Work out the finished part from the listing and answer in its coordinate system (mm). A direction names the side the tool comes from. Coordinates: 2 decimals unless noted, no trailing zeros. Order: outer loops, then holes, each group sorted by start corner. A loop starts at its lowest first (then second) coordinate and runs counter-clockwise, first axis right, second up. Notation, with made-up numbers: (-31.5, 73) - (13.5, 73) arc R19 ccw to (13.5, 92) - close; hole circle Ø6 at (75, -7.5). An arc over 180 degrees is marked (long way). Answer as a JSON object with one key per item and string values. Group by question number.
1) Each of these flat-tipped pins is pushed along its axis until it touches: P1, Ø1.8, axis at x = 29.5, z = -12.5, coming from the +Y side; P2, Ø1.1, axis at y = 2, z = -11, coming from the +X side; P3, Ø3.5, axis at x = -23.5, z = 5, coming from the +Y side; P4, Ø1.5, axis at x = -23.5, y = 1.5, coming from the +Z side. Where does it stop, or does it pass through?
2) Section D-D (z = -12.5) is taken. Give the vertices of the cut face in (x, y), plus the area to 3 significant figures.
3) Section A-A (z = -5) is taken. Give the vertices of the cut face in (x, y).
4) Section B-B (x = -8.5) is taken. Give the vertices of the cut face in (y, z).
5) Section C-C (y = 2.25) is taken. Count the separate pieces of the cut face and the enclosed holes in it, plus the area to 3 significant figures.
6) Find the intervals of material crossed by line 1 along X through (y, z) = (1.45, -5); line 2 along X through (y, z) = (1.3, -12.5); line 3 along X through (y, z) = (3.2, 11.5), in increasing order.
7) A tool of negligible diameter and unlimited length cuts with its end or side. For faces 1 (the face through (-14, 2, 8.5)), 2 (the face through (32.719, 1.521, 15.094)), 3 (the face through (29.5, 1, 0)), 4 (the face through (-25, 2, 1.5)), 5 (the face through (5.6, 3.5, 10)), from which of +Z, -Z, +X, -X, +Y, -Y can it reach the whole face along a straight path? Write none if from no direction.
from build123d import *

# Parameters (mm, degrees)
SKETCH_1_R          = 1.5
SKETCH_1_W          = 24
SKETCH_1_H          = 15
EXTRUDE_1_DEPTH     = 3
SKETCH_2_R          = 2.5
SKETCH_2_R_2        = 1.5
EXTRUDE_2_DEPTH     = 1
CUT_EXTRUDE_1_REACH = 41.246
SKETCH_3_W          = 7
SKETCH_3_H          = 3
FILLET_1_R          = 8
EXTRUDE_3_DEPTH     = 3
CUT_EXTRUDE_2_REACH = 41.246
SKETCH_5_R          = 1.5
EXTRUDE_START       = -3
SKETCH_6_R          = 1.5
EXTRUDE_4_DEPTH     = 3
CUT_EXTRUDE_3_DEPTH = 40.246018906
FILLET_2_R          = 3


with BuildPart() as part:
    # 草图1 → 凸台-拉伸1 (new body)
    with BuildSketch(Plane(origin=(0, 0, 0), x_dir=(1, 0, 0), z_dir=(0, 1, 0))):
        Polygon((-14, -8.5), (0, -8.5), (0, -17.5), (35, -17.5), (35, 17.5), (0, 17.5), (0, 8.5), (-14, 8.5), (-21, 8.5), (-21, -8.5), align=None)
        with Locations(Location((-2.5, 0, 0), (0, 0, 270))):
            Circle(SKETCH_1_R, mode=Mode.SUBTRACT)
        with Locations(Location((29.5, -12.5, 0), (0, 0, 270))):
            Circle(SKETCH_1_R, mode=Mode.SUBTRACT)
        with Locations(Location((5.5, -12.5, 0), (0, 0, 270))):
            Circle(SKETCH_1_R, mode=Mode.SUBTRACT)
        with Locations(Location((29.5, 12.5, 0), (0, 0, 270))):
            Circle(SKETCH_1_R, mode=Mode.SUBTRACT)
        with Locations(Location((5.5, 12.5, 0), (0, 0, 270))):
            Circle(SKETCH_1_R, mode=Mode.SUBTRACT)
        with Locations(Location((-17.5, -5, 0), (0, 0, 270))):
            Circle(SKETCH_1_R, mode=Mode.SUBTRACT)
        with Locations(Location((-17.5, 5, 0), (0, 0, 270))):
            Circle(SKETCH_1_R, mode=Mode.SUBTRACT)
        with Locations((17.5, 0)):
            Rectangle(SKETCH_1_W, SKETCH_1_H, mode=Mode.SUBTRACT)
    extrude(amount=EXTRUDE_1_DEPTH)

    # 草图2 → 凸台-拉伸2 (add)
    # profile 1 of 4: a face of its own
    with BuildSketch(Plane(origin=(0, 3, 0), x_dir=(1, 0, 0), z_dir=(0, 1, 0))):
        with Locations(Location((5.5, 12.5, 0), (0, 0, 270))):
            Circle(SKETCH_2_R)
        with Locations(Location((5.5, 12.5, 0), (0, 0, 270))):
            Circle(SKETCH_2_R_2, mode=Mode.SUBTRACT)
    # profile 2 of 4: a face of its own
    with BuildSketch(Plane(origin=(0, 3, 0), x_dir=(1, 0, 0), z_dir=(0, 1, 0))):
        with Locations(Location((29.5, 12.5, 0), (0, 0, 270))):
            Circle(SKETCH_2_R)
        with Locations(Location((29.5, 12.5, 0), (0, 0, 270))):
            Circle(SKETCH_2_R_2, mode=Mode.SUBTRACT)
    # profile 3 of 4: a face of its own
    with BuildSketch(Plane(origin=(0, 3, 0), x_dir=(1, 0, 0), z_dir=(0, 1, 0))):
        with Locations(Location((29.5, -12.5, 0), (0, 0, 270))):
            Circle(SKETCH_2_R)
        with Locations(Location((29.5, -12.5, 0), (0, 0, 270))):
            Circle(SKETCH_2_R_2, mode=Mode.SUBTRACT)
    # profile 4 of 4: a face of its own
    with BuildSketch(Plane(origin=(0, 3, 0), x_dir=(1, 0, 0), z_dir=(0, 1, 0))):
        with Locations(Location((5.5, -12.5, 0), (0, 0, 270))):
            Circle(SKETCH_2_R)
        with Locations(Location((5.5, -12.5, 0), (0, 0, 270))):
            Circle(SKETCH_2_R_2, mode=Mode.SUBTRACT)
    extrude(amount=EXTRUDE_2_DEPTH)

    # 草图3 → 切除-拉伸1 (cut, up to next)
    with BuildSketch(Plane(origin=(0, 3, 0), x_dir=(1, 0, 0), z_dir=(0, 1, 0)), mode=Mode.PRIVATE) as cut_extrude_1_sk1:
        with Locations((-17.5, 0)):
            Rectangle(SKETCH_3_W, SKETCH_3_H)
    cut_extrude_1_tool1 = extrude(cut_extrude_1_sk1.sketch, amount=-CUT_EXTRUDE_1_REACH, mode=Mode.PRIVATE) & part.part
    add(cut_extrude_1_tool1.solids().sort_by_distance((-17.5, 3, 0))[0], mode=Mode.SUBTRACT)

    # 圆角1
    fillet_1_edges = [part.edges().sort_by_distance(p)[0] for p in [
        (0, 1.5, -17.5),
        (35, 1.5, -17.5),
        (35, 1.5, 17.5),
        (0, 1.5, 17.5),
    ]]
    fillet(fillet_1_edges, radius=FILLET_1_R)

    # 草图4 → 凸台-拉伸3 (add)
    with BuildSketch(Plane(origin=(0, 3, 0), x_dir=(1, 0, 0), z_dir=(0, 1, 0))):
        Polygon((-21, 8.5), (-27, 8.5), (-27, 1.5), (-22.2, 1.5), (-22.2, -1.5), (-27, -1.5), (-27, -8.5), (-21, -8.5), (-21, -1.5), (-14, -1.5), (-14, 1.5), (-21, 1.5), align=None)
    extrude(amount=-EXTRUDE_3_DEPTH)

    # 草图5 → 切除-拉伸2 (cut, up to next)
    with BuildSketch(Plane(origin=(0, 3, 0), x_dir=(1, 0, 0), z_dir=(0, 1, 0)), mode=Mode.PRIVATE) as cut_extrude_2_sk1:
        with Locations(Location((-23.5, 5, 0), (0, 0, 270))):
            Circle(SKETCH_5_R)
    cut_extrude_2_tool1 = extrude(cut_extrude_2_sk1.sketch, amount=-CUT_EXTRUDE_2_REACH, mode=Mode.PRIVATE) & part.part
    # 草图5 → 切除-拉伸2 (cut, up to next)
    with BuildSketch(Plane(origin=(0, 3, 0), x_dir=(1, 0, 0), z_dir=(0, 1, 0)), mode=Mode.PRIVATE) as cut_extrude_2_sk2:
        with Locations(Location((-23.5, -5, 0), (0, 0, 270))):
            Circle(SKETCH_5_R)
    cut_extrude_2_tool2 = extrude(cut_extrude_2_sk2.sketch, amount=-CUT_EXTRUDE_2_REACH, mode=Mode.PRIVATE) & part.part
    # 草图5 → 切除-拉伸2 (cut, up to next)
    with BuildSketch(Plane(origin=(0, 3, 0), x_dir=(1, 0, 0), z_dir=(0, 1, 0)), mode=Mode.PRIVATE) as cut_extrude_2_sk3:
        with Locations(Location((-8.5, 0, 0), (0, 0, 270))):
            Circle(SKETCH_5_R)
    cut_extrude_2_tool3 = extrude(cut_extrude_2_sk3.sketch, amount=-CUT_EXTRUDE_2_REACH, mode=Mode.PRIVATE) & part.part
    add(cut_extrude_2_tool1.solids().sort_by_distance((-23.5, 3, -5))[0], mode=Mode.SUBTRACT)
    add(cut_extrude_2_tool2.solids().sort_by_distance((-23.5, 3, 5))[0], mode=Mode.SUBTRACT)
    add(cut_extrude_2_tool3.solids().sort_by_distance((-8.5, 3, 0))[0], mode=Mode.SUBTRACT)

    # 草图6 → 凸台-拉伸4 (add)
    with BuildSketch(Plane(origin=(0, 3, 0), x_dir=(1, 0, 0), z_dir=(0, 1, 0)).offset(EXTRUDE_START)):
        with Locations((-17.5, 5)):
            Circle(SKETCH_6_R)
        with Locations((-2.5, 0)):
            Circle(SKETCH_6_R)
        with Locations((-17.5, -5)):
            Circle(SKETCH_6_R)
    extrude(amount=EXTRUDE_4_DEPTH)

    # 草图7 → 切除-拉伸3 (cut, through all)
    with BuildSketch(Plane(origin=(0, 3, 0), x_dir=(1, 0, 0), z_dir=(0, 1, 0))):
        Polygon((17.5, 11.5), (12.5, 11.5), (12.5, 7.5), (22.5, 7.5), (22.5, 11.5), align=None)
        Polygon((22.5, -11.5), (17.5, -11.5), (12.5, -11.5), (12.5, -7.5), (22.5, -7.5), align=None)
    extrude(amount=-CUT_EXTRUDE_3_DEPTH, mode=Mode.SUBTRACT)

    # 圆角2
    fillet_2_edges = [part.edges().sort_by_distance(p)[0] for p in [
        (22.5, 1.5, -7.5),
        (12.5, 1.5, -7.5),
        (22.5, 1.5, 7.5),
        (12.5, 1.5, 7.5),
    ]]
    fillet(fillet_2_edges, radius=FILLET_2_R)


solid = part.part
Report:
{
 "1": {"P1": "passes through", "P2": "stops at x = 34.94", "P3": "stops at y = 3", "P4": "stops at z = 8.5"},
 "2": {"outline": "(0.58, 0) - (4, 0) - (4, 4) - (3, 4) - (3, 3) - (0.58, 3) - close; (7, 0) - (28, 0) - (28, 4) - (27, 4) - (27, 3) - (8, 3) - (8, 4) - (7, 4) - close; (31, 0) - (34.42, 0) - (34.42, 3) - (32, 3) - (32, 4) - (31, 4) - close", "area": "87.5 mm²"},
 "3": {"outline": "(-27, 0) - (-25, 0) - (-25, 3) - (-27, 3) - close; (-22, 0) - (5.5, 0) - (5.5, 3) - (-22, 3) - close; (29.5, 0) - (35, 0) - (35, 3) - (29.5, 3) - close"},
 "4": {"outline": "(0, -8.5) - (3, -8.5) - (3, -1.5) - (0, -1.5) - close; (0, 1.5) - (3, 1.5) - (3, 8.5) - (0, 8.5) - close"},
 "5": {"separate pieces": "1", "enclosed holes": "8", "area": "1,120 mm²"},
 "6": {"line 1": "x = -27 to -25, -22 to 5.5, 29.5 to 35", "line 2": "x = 0.58 to 4, 7 to 28, 31 to 34.42", "line 3": "x = 3.21 to 4.38, 6.62 to 7.79, 27.21 to 28.38, 30.62 to 31.79"},
 "7": {"face 1": "+Z, -X, +Y, -Y", "face 2": "+Z, +X, +Y, -Y", "face 3": "+Y, -Y", "face 4": "-X, +Y, -Y", "face 5": "+Y"}
}
